For this review, take the finished solid that the model builds, in its own axes (mm). Face numbers are marked on the shaded views. A direction names the side the tool comes from. Round coordinates to 2 decimals unless told otherwise and drop trailing zeros. Write each loop counter-clockwise with the first axis right and the second up, starting at its lowest first coordinate (ties: lowest second). Pieces come first, ordered by that corner, then holes.
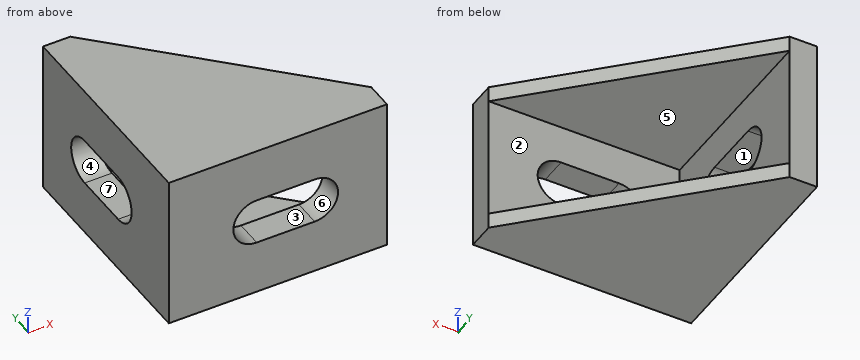
from build123d import *

# Parameters (mm, degrees)
SKETCH1_W           = 20
SKETCH1_H           = 28
BOSS_EXTRUDE1_DEPTH = 3.5
SKETCH2_W           = 20
SKETCH2_H           = 3.5
BOSS_EXTRUDE2_DEPTH = 24.5
BOSS_EXTRUDE3_DEPTH = 2
BOSS_EXTRUDE4_DEPTH = 2
CUT_EXTRUDE1_DEPTH  = 43.240383521
CUT_EXTRUDE2_DEPTH  = 43.240383521


with BuildPart() as part:
    # Sketch1 → Boss-Extrude1 (new body)
    with BuildSketch(Plane(origin=(0, 0, 0), x_dir=(0, 0, -1), z_dir=(1, 0, 0))):
        with Locations((10, 14)):
            Rectangle(SKETCH1_W, SKETCH1_H)
    extrude(amount=BOSS_EXTRUDE1_DEPTH)

    # Sketch2 → Boss-Extrude2 (add)
    with BuildSketch(Plane(origin=(3.5, 0, 0), x_dir=(0, 0, -1), z_dir=(1, 0, 0))):
        with Locations((10, 1.75)):
            Rectangle(SKETCH2_W, SKETCH2_H)
    extrude(amount=BOSS_EXTRUDE2_DEPTH)

    # Sketch3 → Boss-Extrude3 (add)
    with BuildSketch(Plane(origin=(0, 0, -20), x_dir=(-1, 0, 0), z_dir=(0, 0, -1))):
        Polygon((-28, 0), (-28, 3.5), (-3.5, 28), (0, 28), (0, 0), align=None)
    extrude(amount=-BOSS_EXTRUDE3_DEPTH)

    # Sketch4 → Boss-Extrude4 (add)
    with BuildSketch(Plane.XY):
        Polygon((3.5, 28), (0, 28), (0, 0), (28, 0), (28, 3.5), align=None)
    extrude(amount=-BOSS_EXTRUDE4_DEPTH)

    # Sketch5 → Cut-Extrude1 (cut, through all)
    with BuildSketch(Plane(origin=(0, 3.5, 0), x_dir=(1, 0, 0), z_dir=(0, 1, 0))):
        with BuildLine():
            Line((18.718782713, 7), (11.281217287, 7))
            ThreePointArc((11.281217287, 7), (8.281217287, 10), (11.281217287, 13))
            Line((11.281217287, 13), (18.718782713, 13))
            ThreePointArc((18.718782713, 13), (21.718782713, 10), (18.718782713, 7))
        make_face()
    extrude(amount=-CUT_EXTRUDE1_DEPTH, mode=Mode.SUBTRACT)

    # Sketch6 → Cut-Extrude2 (cut, through all)
    with BuildSketch(Plane(origin=(3.5, 0, 0), x_dir=(0, 0, -1), z_dir=(1, 0, 0))):
        with BuildLine():
            Line((7, 11.28), (7, 18.72))
            ThreePointArc((7, 18.72), (10, 21.72), (13, 18.72))
            Line((13, 18.72), (13, 11.28))
            ThreePointArc((13, 11.28), (10, 8.28), (7, 11.28))
        make_face()
    extrude(amount=-CUT_EXTRUDE2_DEPTH, mode=Mode.SUBTRACT)


solid = part.part
(1) For line 1 along Z through (x, y) = (6, 11.25); line 2 along Z through (x, y) = (16.75, 2.5); line 3 along Y through (x, z) = (10.75, -13.5), list the stretches that pass through material, from the lowest coordinate up.
Geometry check:
line 1: z = -20 to -18, -2 to 0
line 2: z = -20 to -13, -7 to 0
line 3: y = 0 to 3.5
(2) For pin 1 Ø4 at (x, z) = (18.5, -5.5) entering from +Y; pin 2 Ø1.5 at (y, z) = (22, -11.5) entering from +X, all flat-tipped, find the tip position at first contact; note any pin that passes through.
Geometry check:
pin 1: stops at y = 3.5
pin 2: stops at x = 3.5
(3) We need section A-A, the plane x = 14.75. Give the boundary of the cut face in (y, z).
Geometry check:
outline: (0, -20) - (16.75, -20) - (16.75, -18) - (3.5, -18) - (3.5, -13) - (0, -13) - close; (0, -7) - (3.5, -7) - (3.5, -2) - (16.75, -2) - (16.75, 0) - (0, 0) - close
(4) We need section B-B, the plane z = -10. Give the boundary of the cut face in (x, y), and give its area (3 significant figures).
Geometry check:
outline: (0, 0) - (8.28, 0) - (8.28, 3.5) - (3.5, 3.5) - (3.5, 8.28) - (0, 8.28) - close; (0, 21.72) - (3.5, 21.72) - (3.5, 28) - (0, 28) - close; (21.72, 0) - (28, 0) - (28, 3.5) - (21.72, 3.5) - close
area: 89.7 mm2
(5) Mouldability with a two-part tool opening along Y and no side actions: class the marked faces 1, 2, 3 and 4 as pulls with the +Y half, pulls with the -Y half, needs draft (parallel to the pull), parting line crosses it, or undercut.
Geometry check:
face 1: undercut
face 2: pulls with the +Y half
face 3: needs draft
face 4: undercut
(6) For the marked faces 5, 6 and 7, list the 3-axis set-ups (+Z, -Z, +X, -X, +Y, -Y) from which the entire face can be reached by the end or side of a thin tool; tool diameter is ignored.
Geometry check:
face 5: +X, +Y
face 6: +Y, -Y
face 7: +X, -X
(7) We need section D-D, the plane y = 10.75. Give the boundary of the cut face in (x, z).
Geometry check:
outline: (0, -20) - (20.75, -20) - (20.75, -18) - (3.5, -18) - (3.5, -12.95) - (0, -12.95) - close; (0, -7.05) - (3.5, -7.05) - (3.5, -2) - (20.75, -2) - (20.75, 0) - (0, 0) - close
(8) We need section C-C, the plane x = 22.5. Give the boundary of the cut face in (y, z), and give its area (3 significant figures).
Geometry check:
outline: (0, -20) - (9, -20) - (9, -18) - (3.5, -18) - (3.5, -2) - (9, -2) - (9, 0) - (0, 0) - close
area: 92.0 mm2
